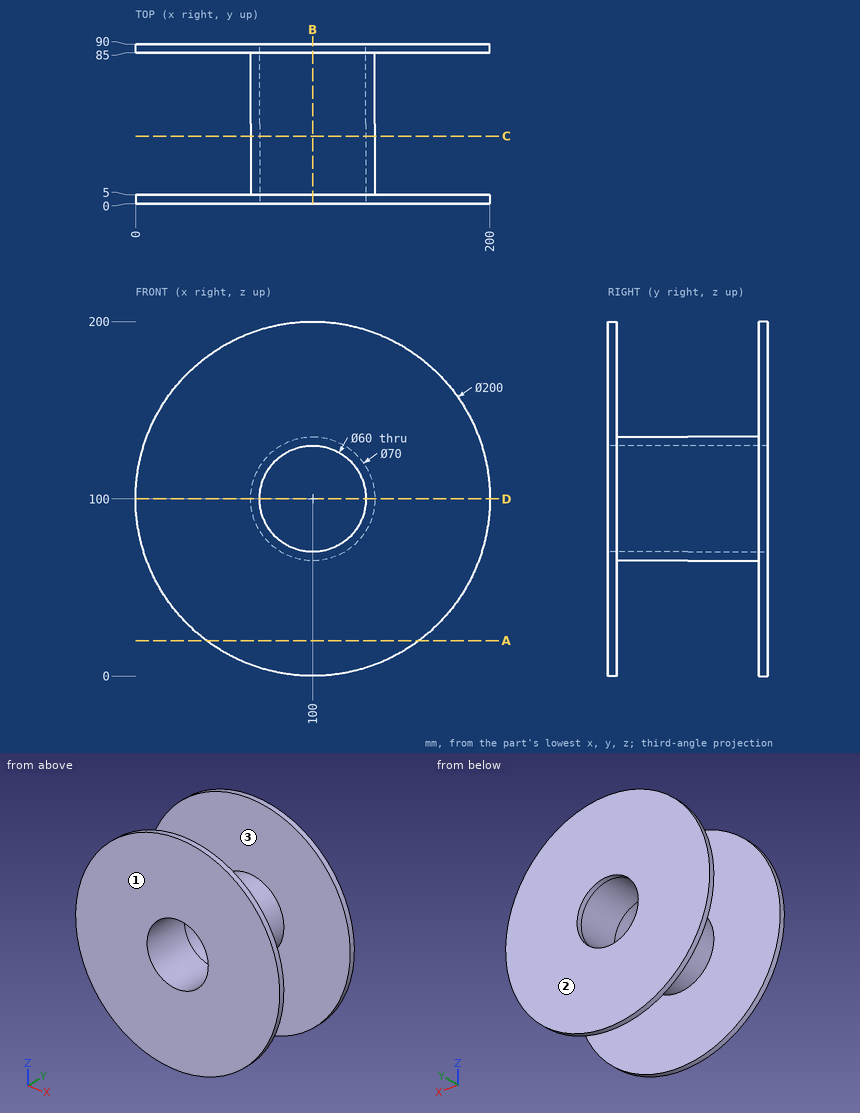
Check sheet for the drawn part. Datum: minimum x, y, z corner. Units: mm. Give positions to 0.01 mm unless a question says otherwise; leave off trailing zeros. Order: outer loops, then holes, each group sorted by start corner. A loop starts at its lowest first (then second) coordinate and runs counter-clockwise, first axis right, second up. Notation, with made-up numbers: (89.25, -12.75) - (145.25, -12.75) arc R24 ccw to (145.25, 7.25) - close; hole circle Ø6 at (20.5, 45.5). An arc over 180 degrees is marked (long way). Write item = value, one per line. Start each with the question number.
1) Section check B-B (x = 100). Enter the section's corners in (y, z).
2) Gauge pin test, flat ends, axial feed: pin 1 Ø2 at (y, z) = (59, 128.5) entering from +X; pin 2 Ø12 at (x, z) = (176, 80.5) entering from -Y; pin 3 Ø3 at (y, z) = (72, 131.5) entering from +X. Record the tip position at first contact, or that the pin passes through.
3) Section check A-A (z = 20). Enter the section's corners in (x, y).
4) Scan lines: L1, parallel to X at y = 57, z = 100; L2, parallel to X at y = 87, z = 100; L3, parallel to Y at x = 188, z = 141.5. Record each from-to range of solid material in increasing order.
5) Section check C-C (y = 38). Enter the section's corners in (x, z), then the cut area to 3 significant figures.
6) Section check D-D (z = 100). Enter the section's corners in (x, y), then the cut area to 3 significant figures.
7) Draft check along Y on the marked faces 1, 2 and 3. Enter one of: released by +Y, released by -Y, zero draft, split by the parting line, or undercut.
Geometry check:
q1.outline = (0, 0) - (5, 0) - (5, 65) - (85, 65) - (85, 0) - (90, 0) - (90, 70) - (0, 70) - close; (0, 130) - (90, 130) - (90, 200) - (85, 200) - (85, 135) - (5, 135) - (5, 200) - (0, 200) - close
q2.pin_1 = 121.65
q2.pin_2 = 0
q2.pin_3 = 118.03
q3.outline = (40, 0) - (160, 0) - (160, 5) - (40, 5) - close; (40, 85) - (160, 85) - (160, 90) - (40, 90) - close
q4.L1 = 65 to 70, 130 to 135
q4.L2 = 0 to 70, 130 to 200
q4.L3 = 0 to 5, 85 to 90
q5.outline = circle Ø70 at (100, 100); hole circle Ø60 at (100, 100)
q5.area = 1,020 mm2
q6.outline = (0, 0) - (70, 0) - (70, 90) - (0, 90) - (0, 85) - (65, 85) - (65, 5) - (0, 5) - close; (130, 0) - (200, 0) - (200, 5) - (135, 5) - (135, 85) - (200, 85) - (200, 90) - (130, 90) - close
q6.area = 2,200 mm2
q7.face_1 = released by -Y
q7.face_2 = released by +Y
q7.face_3 = undercut
